from build123d import *

# Parameters (mm, degrees)
F1_DEPTH = 6
F2_W     = 30
F2_H     = 5.42
F3_DEPTH = 2
F4_R     = 2.25
F5_DEPTH = 8.001
F6_R     = 3.75
F7_DEPTH = 2
F9_DEPTH = 6
F10_SIZE = 3


with BuildPart() as f1:
    # F0 (on Top) → F1 (new body)
    with BuildSketch(Plane.XY):
        Polygon((-40, 0), (-10, 0), (-10, -20), (0, -20), (10, -20), (10, 0), (40, 0), (40, 20), (0, 20), (-40, 20), align=None)
    extrude(amount=F1_DEPTH)

    # F2 (on face) → F3 (join)
    with BuildSketch(Plane.XY.offset(6)):
        Polygon((2.71, 0), (0, 0), (-2.71, 0), (-2.71, -20), (2.71, -20), align=None)
        Polygon((7.845558, 12.71), (7.845558, 10), (7.845558, 7.29), (40, 7.29), (40, 12.71), align=None)
        with Locations((-25, 10)):
            Rectangle(F2_W, F2_H)
    extrude(amount=F3_DEPTH)

    # F4 (on face) → F5 (cut, through all)
    with BuildSketch(Plane(origin=(0, 0, 0), x_dir=(1, 0, 0), z_dir=(0, 0, -1))):
        with Locations((-30, -10)):
            Circle(F4_R)
        with Locations((0, -10)):
            Circle(F4_R)
        with Locations((0, 10)):
            Circle(F4_R)
        with Locations((30, -10)):
            Circle(F4_R)
        with Locations((15, -10)):
            Circle(F4_R)
        with Locations((-15, -10)):
            Circle(F4_R)
    extrude(amount=-F5_DEPTH, mode=Mode.SUBTRACT)

    # F6 (on face) → F7 (cut)
    with BuildSketch(Plane(origin=(0, 0, 0), x_dir=(1, 0, 0), z_dir=(0, 0, -1))):
        with Locations((0, 10)):
            Circle(F6_R)
        with Locations((0, -10)):
            Circle(F6_R)
        with Locations((30, -10)):
            Circle(F6_R)
        with Locations((-30, -10)):
            Circle(F6_R)
        with Locations((-15, -10)):
            Circle(F6_R)
        with Locations((15, -10)):
            Circle(F6_R)
    extrude(amount=-F7_DEPTH, mode=Mode.SUBTRACT)

    # F8 (on face) → F9 (join)
    with BuildSketch(Plane.XY.offset(6)):
        Polygon((-10, 0), (-40, 0), (-10, -20), align=None)
        Polygon((10, 0), (10, -20), (40, 0), align=None)
    extrude(amount=-F9_DEPTH)

    # F10
    f10_edges = [f1.edges().sort_by_distance(p)[0] for p in [
        (-25, -10, 0),
        (0, -20, 0),
        (25, -10, 0),
        (40, 10, 0),
        (-40, 10, 0),
        (0, 20, 0),
    ]]
    chamfer(f10_edges, length=F10_SIZE)


solid = f1.part
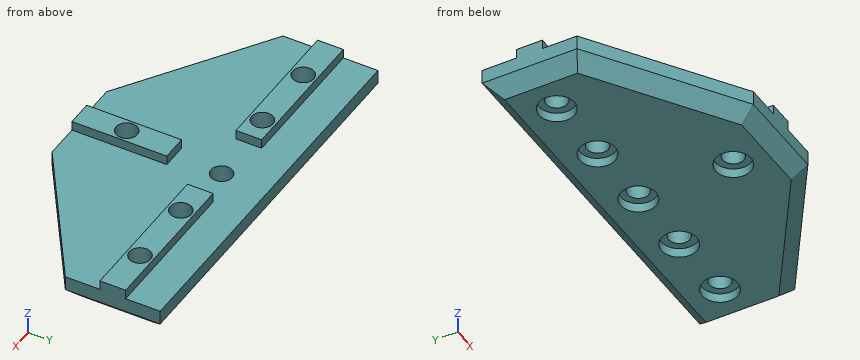
Geometry check sheet. Reference: the model listing, model coordinates, mm. Coordinates: 2 decimals unless noted, no trailing zeros. Order: outer loops, then holes, each group sorted by start corner. A loop starts at its lowest first (then second) coordinate and runs counter-clockwise, first axis right, second up. Notation, with made-up numbers: (-22, 43.5) - (20, 43.5) arc R27 cw to (20, 79.5) - close; hole circle Ø10 at (12.25, -32.75). An arc over 180 degrees is marked (long way). Answer in a Markdown table with one row per item. Add a question column.
1) Cross-section at D-D, the plane x = -15. Record the cut outline in (y, z).
2) Cross-section at A-A, the plane z = 6.75. Record the cut outline in (x, y).
3) Material ranges on line 1 along X through (y, z) = (10, 4.1); line 2 along Y through (x, z) = (0, 4.5); line 3 along X through (y, z) = (10, 1.05), recorded low to high. Write a range as [from, to].
4) Cross-section at B-B, the plane x = 0. Record the cut outline in (y, z).
5) Cross-section at C-C, the plane y = -10. Record the cut outline in (x, z), then the cut area to 3 significant figures.
6) Gauge pin test, flat ends, axial feed: P1, Ø10, axis at x = 15, y = 10, coming from the -Z side; P2, Ø5, axis at x = 15, y = 10, coming from the -Z side; P3, Ø1, axis at y = -7, z = 7.5, coming from the -X side; P4, Ø4, axis at y = -2.5, z = 4, coming from the -X side. Record the tip position at first contact, or that the pin passes through.
Check result:
| question | item | result |
|---|---|---|
| 1 | outline | (-16.67, 3) - (-13.06, 0) - (6.25, 0) - (6.25, 2) - (7.75, 2) - (7.75, 8) - (7.29, 8) - (7.29, 6) - (-16.67, 6) - close; (12.25, 2) - (13.75, 2) - (13.75, 0) - (17, 0) - (20, 3) - (20, 6) - (12.71, 6) - (12.71, 8) - (12.25, 8) - close |
| 2 | outline | (-40, 7.29) - (-10, 7.29) - (-10, 12.71) - (-40, 12.71) - close; (-2.71, -20) - (2.71, -20) - (2.71, 0) - (-2.71, 0) - close; (7.85, 7.29) - (40, 7.29) - (40, 12.71) - (7.85, 12.71) - close; hole circle Ø4.5 at (-30, 10); hole circle Ø4.5 at (-15, 10); hole circle Ø4.5 at (0, -10); hole circle Ø4.5 at (15, 10); hole circle Ø4.5 at (30, 10) |
| 3 | line 1 | x = [-40, -32.25], [-27.75, -17.25], [-12.75, -2.25], [2.25, 12.75], [17.25, 27.75], [32.25, 40] |
| 3 | line 2 | y = [-20, -12.25], [-7.75, 7.75], [12.25, 20] |
| 3 | line 3 | x = [-38.05, -33.75], [-26.25, -18.75], [-11.25, -3.75], [3.75, 11.25], [18.75, 26.25], [33.75, 38.05] |
| 4 | outline | (-20, 3) - (-17, 0) - (-13.75, 0) - (-13.75, 2) - (-12.25, 2) - (-12.25, 8) - (-20, 8) - close; (-7.75, 2) - (-6.25, 2) - (-6.25, 0) - (6.25, 0) - (6.25, 2) - (7.75, 2) - (7.75, 6) - (0, 6) - (0, 8) - (-7.75, 8) - close; (12.25, 2) - (13.75, 2) - (13.75, 0) - (17, 0) - (20, 3) - (20, 6) - (12.25, 6) - close |
| 5 | outline | (-25, 3) - (-19.59, 0) - (-3.75, 0) - (-3.75, 2) - (-2.25, 2) - (-2.25, 8) - (-2.71, 8) - (-2.71, 6) - (-25, 6) - close; (2.25, 2) - (3.75, 2) - (3.75, 0) - (19.59, 0) - (25, 3) - (25, 6) - (2.71, 6) - (2.71, 8) - (2.25, 8) - close |
| 5 | area | 253 mm² |
| 6 | P1 | stops at z = 0 |
| 6 | P2 | stops at z = 2 |
| 6 | P3 | stops at x = -2.71 |
| 6 | P4 | stops at x = -39.25 |
